```python
from build123d import *

# Parameters (mm, degrees)
SKETCH_2_R      = 2
EXTRUDE_2_DEPTH = 5
SKETCH_4_W      = 50
SKETCH_4_H      = 5
EXTRUDE_3_DEPTH = 10


with BuildPart() as part:
    # 草图2 → 凸台-拉伸2 (new body)
    with BuildSketch(Plane(origin=(0, 0, 0), x_dir=(0, 0, -1), z_dir=(1, 0, 0))):
        with BuildLine():
            Line((-25, 9.903100775), (-10.246516239, 9.903100775))
            ThreePointArc((-10.246516239, 9.903100775), (0, -14.25), (10.246516239, 9.903100775))
            Line((10.246516239, 9.903100775), (25, 9.903100775))
            Line((25, 9.903100775), (25, -43.166899225))
            Line((25, -43.166899225), (-25, -43.166899225))
            Line((-25, -43.166899225), (-25, 9.903100775))
        make_face()
        with Locations((17.5, 0)):
            Circle(SKETCH_2_R, mode=Mode.SUBTRACT)
        with Locations((-17.5, 0)):
            Circle(SKETCH_2_R, mode=Mode.SUBTRACT)
    extrude(amount=EXTRUDE_2_DEPTH)

    # 草图4 → 凸台-拉伸3 (add)
    with BuildSketch(Plane.ZY):
        with Locations((0, -40.666899225)):
            Rectangle(SKETCH_4_W, SKETCH_4_H)
    extrude(amount=EXTRUDE_3_DEPTH)


solid = part.part
```
The listing builds one solid part. Answer for the finished solid, in the listing's coordinates (mm). A direction names the side the tool comes from. Round coordinates to 2 decimals unless told otherwise and drop trailing zeros. Order: outer loops, then holes, each group sorted by start corner. A loop starts at its lowest first (then second) coordinate and runs counter-clockwise, first axis right, second up. Notation, with made-up numbers: (-39, -26) - (-35, -26) arc R11 ccw to (-35, -12) - close; hole circle Ø9 at (6.5, -19.75). An arc over 180 degrees is marked (long way). Put each result on its own line as item: value. Start each with the question number.
(1) Straight lines are drawn through the part: probe 1 along Y at (x, z) = (3.2, 17.5); probe 2 along Y at (x, z) = (-3.5, -15); probe 3 along X at (y, z) = (-27, -9). For each, find the intervals that lie inside material, in ascending order. Write a range as from..to.
(2) Find section A-A (y = 0). Give the vertices of the cut face in (x, z), plus the area to 3 significant figures.
(3) Given P1, Ø3, axis at x = -4, z = 3, coming from the +Y side; P2, Ø10, axis at y = -7.5, z = -4, coming from the +X side; P3, Ø14.5, axis at y = -12.5, z = -9.5, coming from the -X side, each flat-ended and moving along its own axis, determine where each tip first touches the part or whether it passes through.
(4) Find section B-B (z = -17.5). Give the vertices of the cut face in (x, y), plus the area to 3 significant figures.
(5) Find section C-C (x = 2.25). Give the vertices of the cut face in (y, z), plus the area to 3 significant figures.
(6) Find section D-D (y = -13). Give the vertices of the cut face in (x, z), plus the area to 3 significant figures.
(7) For faces 4 (the flat face through (-2, -43.167, 0)), 5 (the flat face through (0, -19, 0)), determine the directions among +Z, -Z, +X, -X, +Y, -Y from which every point of the face is accessible in a straight line to the end or side of a thin tool.
(8) Determine the mould class of faces 1 (the flat face through (2, 9.903, -18)), 2 (the cylindrical face through (2.465, -14.242, 0.467)), 3 (the flat face through (1, -23, -25)) for opening direction Z: released by +Z, released by -Z, zero draft, split by the parting line, or undercut.
Reply:
1. probe 1: -43.17..-2, 2..9.9
1. probe 2: -43.17..-38.17
1. probe 3: 0..5
2. outline: (0, -25) - (5, -25) - (5, -19.5) - (0, -19.5) - close; (0, -15.5) - (5, -15.5) - (5, -14.25) - (0, -14.25) - close; (0, 14.25) - (5, 14.25) - (5, 15.5) - (0, 15.5) - close; (0, 19.5) - (5, 19.5) - (5, 25) - (0, 25) - close
2. area: 67.5 mm^2
3. P1: y = -38.17
3. P2: through
3. P3: x = 0
4. outline: (-10, -43.17) - (5, -43.17) - (5, -2) - (0, -2) - (0, -38.17) - (-10, -38.17) - close; (0, 2) - (5, 2) - (5, 9.9) - (0, 9.9) - close
4. area: 295 mm^2
5. outline: (-43.17, -25) - (9.9, -25) - (9.9, -10.25) arc R14.25 cw (long way) to (9.9, 10.25) - (9.9, 25) - (-43.17, 25) - close; hole circle Ø4 at (0, -17.5); hole circle Ø4 at (0, 17.5)
5. area: 2,050 mm^2
6. outline: (0, -25) - (5, -25) - (5, -5.84) - (0, -5.84) - close; (0, 5.84) - (5, 5.84) - (5, 25) - (0, 25) - close
6. area: 192 mm^2
7. face 4: +Z, -Z, +X, -X, -Y
7. face 5: +Z, -Z, -X, +Y
8. face 1: zero draft
8. face 2: undercut
8. face 3: released by -Z
